Work out the finished part from the listing and answer in its coordinate system (mm). Face numbers are marked on the shaded views. A direction names the side the tool comes from. Round coordinates to 2 decimals unless told otherwise and drop trailing zeros. Loops run counter-clockwise (first coordinate to the right, second up) from the corner with the lowest first, then second, coordinate; pieces in that order, holes last. Notation, with made-up numbers: (52.5, -18) - (65.5, -18) arc R24 ccw to (65.5, 9) - close; hole circle Ø9 at (60.25, 67). An arc over 180 degrees is marked (long way). Use CSV: the item, a comma, the result in double quotes. Start each with the question number.
from build123d import *

# Parameters (mm, degrees)
SKETCH1_R           = 11
BOSS_EXTRUDE1_DEPTH = 3.5
SKETCH3_R           = 3.5
CUT_EXTRUDE1_DEPTH  = 8
SKETCH3_3_R         = 8.75
SKETCH3_3_R_2       = 5.75
CUT_EXTRUDE2_DEPTH  = 1.8
FILLET1_R           = 0.5


with BuildPart() as part:
    # Sketch1 → Boss-Extrude1 (new body, symmetric)
    with BuildSketch(Plane(origin=(0, 0, 0), x_dir=(1, 0, 0), z_dir=(0, 1, 0))):
        Circle(SKETCH1_R)
    extrude(amount=BOSS_EXTRUDE1_DEPTH, both=True)

    # Sketch3 → Cut-Extrude1 (cut, through all)
    with BuildSketch(Plane(origin=(0, 3.5, 0), x_dir=(1, 0, 0), z_dir=(0, 1, 0))):
        Circle(SKETCH3_R)
    extrude(amount=-CUT_EXTRUDE1_DEPTH, mode=Mode.SUBTRACT)

    # Sketch3<3> → Cut-Extrude2 (cut)
    with BuildSketch(Plane(origin=(0, 3.5, 0), x_dir=(1, 0, 0), z_dir=(0, 1, 0))):
        Circle(SKETCH3_3_R)
        Circle(SKETCH3_3_R_2, mode=Mode.SUBTRACT)
    cut_extrude2 = extrude(amount=-CUT_EXTRUDE2_DEPTH, mode=Mode.SUBTRACT)

    # Mirror1: Cut-Extrude2 across plane
    add(cut_extrude2.mirror(Plane.ZX), mode=Mode.SUBTRACT)

    # Fillet1
    fillet1_edges = [part.edges().sort_by_distance(p)[0] for p in [
        (-5.75, 3.5, 0),
        (-11, -3.5, 0),
        (-5.75, -3.5, 0),
        (-11, 3.5, 0),
    ]]
    fillet(fillet1_edges, radius=FILLET1_R)


solid = part.part
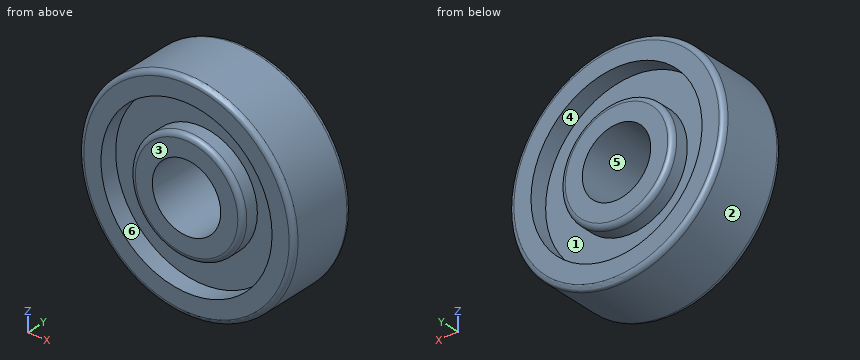
Item 1: Find the intervals of material crossed by probe 1 along Z at (x, y) = (0, 2.65); probe 2 along X at (y, z) = (0.75, 0), in increasing order. Write a range as [from, to].
Item 2: The mould has two halves that part along X. Classify the marked faces 1, 2 and 3: pulls with the +X half, pulls with the -X half, needs draft (parallel to the pull), parting line crosses it, or undercut.
Item 3: Each of these flat-tipped pins is pushed along its axis until it touches: pin 1 Ø3 at (y, z) = (2.5, -7) entering from -X; pin 2 Ø2 at (y, z) = (-1.5, -2.5) entering from -X. Where does it stop, or does it pass through?
Item 4: A cutting plane is placed at C-C (y = 0.25). Determine the outline of the cut face in (x, z), plus the area to 3 significant figures.
Item 5: Which of the six approach directions +Z, -Z, +X, -X, +Y, -Y give full straight-line access (tool end or side, diameter ignored) to the marked faces 4, 5 and 6?
Result sheet:
1,probe 1,"[-11, -8.75], [-5.75, -3.5], [3.5, 5.75], [8.75, 11]"
1,probe 2,"[-11, -3.5], [3.5, 11]"
2,face 1,"undercut"
2,face 2,"parting line crosses it"
2,face 3,"needs draft"
3,pin 1,"x = -9.53"
3,pin 2,"x = -10.9"
4,outline,"circle Ø22 at (0, 0); hole circle Ø7 at (0, 0)"
4,area,"342 mm^2"
5,face 4,"+Y"
5,face 5,"+Y, -Y"
5,face 6,"-Y"
